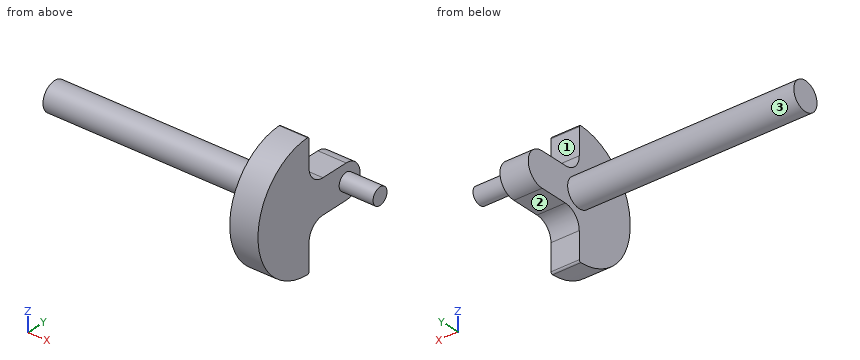
from build123d import *

# Parameters (mm, degrees)
SKETCH2_R           = 1.190625
SKETCH2_R_2         = 1.984375
BOSS_EXTRUDE1_DEPTH = 3.96875
SKETCH3_R           = 1.190625
BOSS_EXTRUDE2_DEPTH = 8.73125
SKETCH4_R           = 1.984375
BOSS_EXTRUDE3_DEPTH = 31.75
SKETCH5_R           = 1.984375
BOSS_EXTRUDE4_DEPTH = 3.96875
FILLET2_R           = 2.38125
FILLET3_R           = 0.254


with BuildPart() as part:
    # Sketch2 → Boss-Extrude1 (new body)
    with BuildSketch(Plane(origin=(0, 0, 0), x_dir=(0, 0, -1), z_dir=(1, 0, 0))):
        with BuildLine():
            Line((8.73125, 0), (2.38125, 0))
            Line((2.38125, 0), (2.38125, 6.35))
            ThreePointArc((2.38125, 6.35), (0, 8.73125), (-2.38125, 6.35))
            Line((-2.38125, 6.35), (-2.38125, 0))
            Line((-2.38125, 0), (-8.73125, 0))
            ThreePointArc((-8.73125, 0), (0, -8.73125), (8.73125, 0))
        make_face()
        with Locations((0, 6.35)):
            Circle(SKETCH2_R, mode=Mode.SUBTRACT)
        Circle(SKETCH2_R_2, mode=Mode.SUBTRACT)
    extrude(amount=BOSS_EXTRUDE1_DEPTH)

    # Sketch3 → Boss-Extrude2 (add)
    with BuildSketch(Plane.ZY):
        with Locations((0, 6.35)):
            Circle(SKETCH3_R)
    extrude(amount=-BOSS_EXTRUDE2_DEPTH)



with BuildPart() as body_2:
    # Sketch4 → Boss-Extrude3 (new body)
    with BuildSketch(Plane.ZY):
        Circle(SKETCH4_R)
    extrude(amount=BOSS_EXTRUDE3_DEPTH)


with BuildPart() as part_1:
    add(part.part)

    add(body_2.part)  # Boss-Extrude4 merges body 2
    # Sketch5 → Boss-Extrude4 (add)
    with BuildSketch(Plane(origin=(0, 0, 0), x_dir=(0, 0, -1), z_dir=(1, 0, 0))):
        Circle(SKETCH5_R)
    extrude(amount=BOSS_EXTRUDE4_DEPTH)

    # Fillet2
    fillet2_edges = [part_1.edges().sort_by_distance(p)[0] for p in [
        (1.984375, 0, -2.38125),
        (1.984375, 0, 2.38125),
    ]]
    fillet(fillet2_edges, radius=FILLET2_R)

    # Fillet3
    fillet3_edges = [part_1.edges().sort_by_distance(p)[0] for p in [
        (1.984375, 0, -8.73125),
        (1.984375, 0, 8.73125),
    ]]
    fillet(fillet3_edges, radius=FILLET3_R)


solid = part_1.part
The model under review builds one solid part; all positions refer to its coordinate system, in mm. Face numbers are marked on the shaded views. A direction names the side the tool comes from. Give positions to 0.01 mm unless a question says otherwise; leave off trailing zeros. Loops run counter-clockwise (first coordinate to the right, second up) from the corner with the lowest first, then second, coordinate; pieces in that order, holes last. Notation, with made-up numbers: (84, -11) -> (113, -11) arc R6 ccw to (113, 0) -> close; hole circle Ø3 at (80.5, 64.25). An arc over 180 degrees is marked (long way). Put each result on its own line as item: value. Start each with the question number.
1. Clearance check with flat-ended pins moving along their axes: P1, Ø2, axis at x = -1.5, z = 1, coming from the -Y side; P2, Ø4, axis at x = -10.5, y = -3, coming from the +Z side; P3, Ø5, axis at y = -3, z = 2.5, coming from the +X side. State where each tip first meets the part, or that it passes through.
2. We need section C-C on x = -12. State the section outline as (y, z) points.
3. We need section B-B on y = 1.5. State the section outline as (x, z) points, then the cut area to 3 significant figures.
4. For the marked faces 1, 2 and 3, list the 3-axis set-ups (+Z, -Z, +X, -X, +Y, -Y) from which the entire face can be reached by the end or side of a thin tool; tool diameter is ignored.
5. We need section D-D on y = -4.25. State the section outline as (x, z) points, then the cut area to 3 significant figures.
6. Wall thickness on probe 1 along X at (y, z) = (7, 0.25); probe 2 along Z at (x, y) = (-1, 0); probe 3 along X at (y, z) = (2.5, -1.25): over which ranges is each line inside the solid? List them lowest first.
7. We need section A-A on z = 0. State the section outline as (x, y) points.
Determined:
1. P1: y = -1.98
1. P2: z = 1.71
1. P3: x = 3.97
2. outline: circle Ø3.97 at (0, 0)
3. outline: (-31.75, -1.3) -> (0, -1.3) -> (0, -2.55) -> (3.97, -2.55) -> (3.97, 2.55) -> (0, 2.55) -> (0, 1.3) -> (-31.75, 1.3) -> close
3. area: 103 mm^2
4. face 1: +Z, +X, -X, +Y
4. face 2: -Z, +X, -X, +Y
4. face 3: -X
5. outline: (0, -7.63) -> (3.97, -7.63) -> (3.97, 7.63) -> (0, 7.63) -> close
5. area: 60.5 mm^2
6. probe 1: 0 to 8.73
6. probe 2: -1.98 to 1.98
6. probe 3: 0 to 3.97
7. outline: (-31.75, -1.98) -> (0, -1.98) -> (0, -8.73) -> (3.97, -8.73) -> (3.97, 5.16) -> (8.73, 5.16) -> (8.73, 7.54) -> (3.97, 7.54) -> (3.97, 8.73) -> (0, 8.73) -> (0, 1.98) -> (-31.75, 1.98) -> close
